Here's how the part is built. I have some questions about the finished solid (model axes, mm). A direction names the side the tool comes from. Coordinates: 2 decimals unless noted, no trailing zeros. Write each loop counter-clockwise with the first axis right and the second up, starting at its lowest first coordinate (ties: lowest second). Pieces come first, ordered by that corner, then holes. Notation, with made-up numbers: (46.25, -33) - (93.25, -33) arc R17 cw to (93.25, -8) - close; hole circle Ø8 at (75, -34.75). An arc over 180 degrees is marked (long way). Answer in a Markdown table with one row per item. Add a question column.
Item 1: Which directions (+Z, -Z, +X, -X, +Y, -Y) give clear straight access to the entire face, cutting with the end or side of a thin tool? Please do faces 4 (the face through (6, 3.4, -3.4)), 5 (the face through (4.58, -1.73, -7.81)), 6 (the face through (2.38, 1.48, 1.46)).
Item 2: I'm going to push flat-ended pins straight in: pin 1 (8 mm diameter, centred on x = 6.5, y = 5.5, fed in from +Z); pin 2 (0.6 mm diameter, centred on y = -0.5, z = -2, fed in from -X); pin 3 (1 mm diameter, centred on x = 9, y = 1.5, fed in from -Z); pin 4 (2 mm diameter, centred on x = 11, y = -6, fed in from +Z). Where does each tip first touch, or does it pass through?
Item 3: If I drill on probe 1 along Y at (x, z) = (9.75, 3.5); probe 2 along Y at (x, z) = (10.25, -1.75); probe 3 along X at (y, z) = (2.25, 4.75), over which ranges is the centre line in solid material (lowest first)? Write a range as from..to.
Item 4: Imagine slicing it at A-A (x = 8). Please give me the cut outline in (y, z), plus the area to 3 significant figures.
Item 5: We'd pull the mould along Z, two halves only. Please class faces 1 (the face through (11.267, -0.867, -3.905)), 2 (the face through (2.604, 0.015, -3.102)), 3 (the face through (16, 0, 0)): +Z half, -Z half, draft (parallel to the pull), parting line (faces both ways), or undercut.
from build123d import *

# Parameters (mm, degrees)
RECPAT_COUNT = 2
RECPAT_ANGLE = 90


with BuildPart() as part:
    # Fillet1: read off the stored shape, not the designer's step
    # Fillet1 outline → Fillet1 (revolve)
    with BuildSketch(Plane.YX):
        with BuildLine():
            Line((4, 6.4), (4, 16))
            Line((4, 16), (0, 16))
            Line((0, 16), (0, 0))
            ThreePointArc((0, 0), (4.055866915, 0.648888974), (7.706840396, 2.530777913))
            ThreePointArc((7.706840396, 2.530777913), (7.922543805, 2.785746454), (8, 3.110611748))
            Line((8, 3.110611748), (8, 6))
            Line((8, 6), (4.4, 6))
            ThreePointArc((4.4, 6), (4.117157288, 6.117157288), (4, 6.4))
        make_face()
    revolve(axis=Axis((0, 0, 0), (1, 0, 0)))

    # Sketch3 → Recess section 0
    with BuildSketch(Plane(origin=(0, 0, 0), x_dir=(0, 0, -1), z_dir=(1, 0, 0))):
        with BuildLine():
            Line((1.08, -4.4), (-1.08, -4.4))
            Line((-1.08, -4.4), (-1.08, 4.4))
            Line((-1.08, 4.4), (1.08, 4.4))
            Line((1.08, 4.4), (1.08, -4.4))
        make_face()
    # Sketch4 → Recess section 1
    with BuildSketch(Plane(origin=(4.5, 0, 0), x_dir=(0, 0, -1), z_dir=(1, 0, 0))):
        with BuildLine():
            Line((1.08, -2.156383139), (-1.08, -2.156383139))
            Line((-1.08, -2.156383139), (-1.08, 2.156383139))
            Line((-1.08, 2.156383139), (1.08, 2.156383139))
            Line((1.08, 2.156383139), (1.08, -2.156383139))
        make_face()
    recess = loft(mode=Mode.SUBTRACT)

    # RecPat: Recess ×2 about axis
    recpat_axis = Axis((0, 0, 0), (1, 0, 0))
    for i in range(1, RECPAT_COUNT):
        add(recess.rotate(recpat_axis, i * RECPAT_ANGLE / (RECPAT_COUNT - 1)), mode=Mode.SUBTRACT)

    # RecCorSke → RecessCore (revolve, cut)
    with BuildSketch(Plane.XY, mode=Mode.PRIVATE) as recesscore_sk:
        Polygon((0, 0), (0, 2.245170654), (4.5, 1.9305), (5.127257474, 0), align=None)
    revolve(recesscore_sk.sketch.rotate(Axis((-3.175, 0, 0), (1, 0, 0)), 90), axis=Axis((-3.175, 0, 0), (1, 0, 0)), mode=Mode.SUBTRACT)


solid = part.part
Here are the results:
| question | item | result |
|---|---|---|
| 1 | face 4 | +X |
| 1 | face 5 | +X, -X |
| 1 | face 6 | -X |
| 2 | pin 1 | stops at z = 7.85 |
| 2 | pin 2 | stops at x = 4.21 |
| 2 | pin 3 | stops at z = -3.87 |
| 2 | pin 4 | passes through |
| 3 | probe 1 | y = -1.94..1.94 |
| 3 | probe 2 | y = -3.6..3.6 |
| 3 | probe 3 | x = 1.11..6 |
| 4 | outline | circle Ø8 at (0, 0) |
| 4 | area | 50.3 mm2 |
| 5 | face 1 | parting line |
| 5 | face 2 | undercut |
| 5 | face 3 | draft |
